Part model, mm, in its own coordinate system. Give positions to 0.01 mm unless a question says otherwise; leave off trailing zeros. Order: outer loops, then holes, each group sorted by start corner. A loop starts at its lowest first (then second) coordinate and runs counter-clockwise, first axis right, second up.
1. Slice it at B-B on z = 14. List the corners of the cut face in (x, y).
2. Drop flat-ended pins along their axis: pin 1 Ø4 at (x, y) = (-5, 2) entering from -Z; pin 2 Ø2 at (y, z) = (5.5, 11) entering from +X; pin 3 Ø1 at (x, z) = (6.5, -16.5) entering from -Y. Give the stop position or say it passes through.
3. Probe line 1 (Z direction, x = 8.5, y = 1.5); line 2 (X direction, y = 9, z = 0.5); line 3 (Z direction, x = -35, y = 1.5). List the from-to ranges inside material, lowest first.
4. Slice it at A-A on y = 2. List the corners of the cut face in (x, z) (1 decimal), and give its area (3 significant figures).
5. Slice it at D-D on x = 26.5. List the corners of the cut face in (y, z), and give its area (3 significant figures).
6. Slice it at C-C on z = -10. List the corners of the cut face in (x, y), and give its area (3 significant figures).
from build123d import *

# Parameters (mm, degrees)
RESSALTO_EXTRUS_O1_DEPTH = 10


with BuildPart() as part:
    # Esboço1 → Ressalto-extrusão1 (new body)
    with BuildSketch(Plane(origin=(0, 0, 0), x_dir=(1, 0, 0), z_dir=(0, 1, 0))):
        with BuildLine():
            ThreePointArc((-39.209518669, -7.912878475), (-38.076880663, -12.253618198), (-36.465309506, -16.440231222))
            ThreePointArc((-36.465309506, -16.440231222), (-33.509440947, -16.163395048), (-31.176914536, -18))
            Line((-31.176914536, -18), (-17.320508076, -10))
            ThreePointArc((-17.320508076, -10), (-17.320508076, 10), (0, 20))
            Line((0, 20), (0, 36))
            ThreePointArc((0, 36), (-2.75680975, 37.101724651), (-3.994996871, 39.8))
            ThreePointArc((-3.994996871, 39.8), (-8.426495684, 39.102355051), (-12.752005558, 37.912878475))
            Line((-12.752005558, 37.912878475), (-39.209518669, -7.912878475))
        make_face()
        with BuildLine():
            Line((-8.660254038, 45), (-12.752005558, 37.912878475))
            ThreePointArc((-12.752005558, 37.912878475), (-8.426495684, 39.102355051), (-3.994996871, 39.8))
            ThreePointArc((-3.994996871, 39.8), (-2.898275349, 42.75680975), (0, 44))
            Line((0, 44), (0, 50))
            ThreePointArc((0, 50), (-5, 48.660254038), (-8.660254038, 45))
        make_face()
        with BuildLine():
            ThreePointArc((8.660254038, 45), (5, 48.660254038), (0, 50))
            Line((0, 50), (0, 44))
            ThreePointArc((0, 44), (2.828427125, 42.828427125), (4, 40))
            ThreePointArc((4, 40), (3.998749022, 39.899968716), (3.994996871, 39.8))
            ThreePointArc((3.994996871, 39.8), (8.426495684, 39.102355051), (12.752005558, 37.912878475))
            Line((12.752005558, 37.912878475), (8.660254038, 45))
        make_face()
        with BuildLine():
            Line((0, 36), (0, 20))
            ThreePointArc((0, 20), (14.142135624, 14.142135624), (20, 0))
            ThreePointArc((20, 0), (19.318516526, -5.176380902), (17.320508076, -10))
            Line((17.320508076, -10), (31.176914536, -18))
            ThreePointArc((31.176914536, -18), (33.509440947, -16.163395048), (36.465309506, -16.440231222))
            ThreePointArc((36.465309506, -16.440231222), (38.076880663, -12.253618198), (39.209518669, -7.912878475))
            Line((39.209518669, -7.912878475), (12.752005558, 37.912878475))
            ThreePointArc((12.752005558, 37.912878475), (8.426495684, 39.102355051), (3.994996871, 39.8))
            ThreePointArc((3.994996871, 39.8), (2.75680975, 37.101724651), (0, 36))
        make_face()
        with BuildLine():
            ThreePointArc((-30.641016151, -20), (-31.127982273, -21.912744878), (-32.470312635, -23.359768778))
            ThreePointArc((-32.470312635, -23.359768778), (-29.65038498, -26.848736852), (-26.457513111, -30))
            Line((-26.457513111, -30), (26.457513111, -30))
            ThreePointArc((26.457513111, -30), (29.65038498, -26.848736852), (32.470312635, -23.359768778))
            ThreePointArc((32.470312635, -23.359768778), (30.752631197, -20.938329603), (31.176914536, -18))
            Line((31.176914536, -18), (17.320508076, -10))
            ThreePointArc((17.320508076, -10), (0, -20), (-17.320508076, -10))
            Line((-17.320508076, -10), (-31.176914536, -18))
            ThreePointArc((-31.176914536, -18), (-30.777312846, -18.96472382), (-30.641016151, -20))
        make_face()
        with BuildLine():
            ThreePointArc((-43.301270189, -15), (-44.641016151, -20), (-43.301270189, -25))
            Line((-43.301270189, -25), (-38.105117767, -22))
            ThreePointArc((-38.105117767, -22), (-38.477621103, -18.868424796), (-36.465309506, -16.440231222))
            ThreePointArc((-36.465309506, -16.440231222), (-38.076880663, -12.253618198), (-39.209518669, -7.912878475))
            Line((-39.209518669, -7.912878475), (-43.301270189, -15))
        make_face()
        with BuildLine():
            Line((-38.105117767, -22), (-43.301270189, -25))
            ThreePointArc((-43.301270189, -25), (-39.641016151, -28.660254038), (-34.641016151, -30))
            Line((-34.641016151, -30), (-26.457513111, -30))
            ThreePointArc((-26.457513111, -30), (-29.65038498, -26.848736852), (-32.470312635, -23.359768778))
            ThreePointArc((-32.470312635, -23.359768778), (-35.579345754, -23.888384955), (-38.105117767, -22))
        make_face()
        with BuildLine():
            Line((38.105117767, -22), (43.301270189, -25))
            ThreePointArc((43.301270189, -25), (44.641016151, -20), (43.301270189, -15))
            Line((43.301270189, -15), (39.209518669, -7.912878475))
            ThreePointArc((39.209518669, -7.912878475), (38.076880663, -12.253618198), (36.465309506, -16.440231222))
            ThreePointArc((36.465309506, -16.440231222), (38.054018746, -17.913995856), (38.641016151, -20))
            ThreePointArc((38.641016151, -20), (38.504719457, -21.03527618), (38.105117767, -22))
        make_face()
        with BuildLine():
            ThreePointArc((32.470312635, -23.359768778), (29.65038498, -26.848736852), (26.457513111, -30))
            Line((26.457513111, -30), (34.641016151, -30))
            ThreePointArc((34.641016151, -30), (39.641016151, -28.660254038), (43.301270189, -25))
            Line((43.301270189, -25), (38.105117767, -22))
            ThreePointArc((38.105117767, -22), (35.579345754, -23.888384955), (32.470312635, -23.359768778))
        make_face()
    extrude(amount=RESSALTO_EXTRUS_O1_DEPTH)


solid = part.part
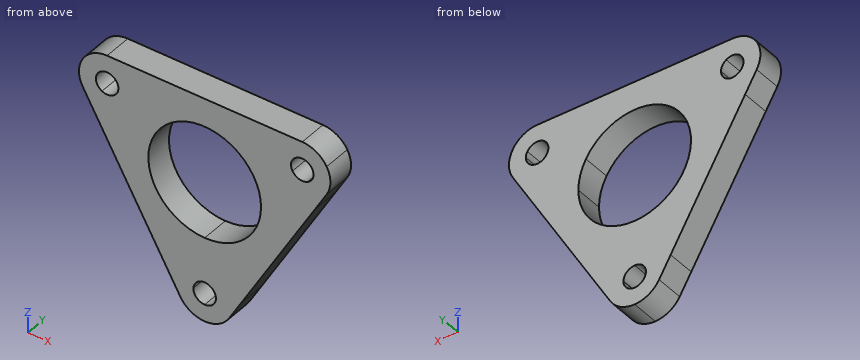
Data:
1. outline: (-42.72, 0) - (-14.28, 0) - (-14.28, 10) - (-42.72, 10) - close; (14.28, 0) - (42.72, 0) - (42.72, 10) - (14.28, 10) - close
2. pin 1: stops at z = -49.54
2. pin 2: stops at x = 41.57
2. pin 3: passes through
3. line 1: z = -45.27 to -18.1, 18.1 to 30
3. line 2: x = -34.93 to -19.99, 19.99 to 34.93
3. line 3: z = 0.62 to 16.02, 23.98 to 29.99
4. outline: (-43.3, 15) - (-8.7, -45) arc R10 ccw to (8.7, -45) - (43.3, 15) arc R10 ccw to (34.6, 30) - (-34.6, 30) arc R10 ccw to start; hole circle Ø8 at (-34.6, 20); hole circle Ø40 at (0, 0); hole circle Ø8 at (0, -40); hole circle Ø8 at (34.6, 20)
4. area: 3,060 mm2
5. outline: (0, -14.1) - (10, -14.1) - (10, 30) - (0, 30) - close
5. area: 441 mm2
6. outline: (-28.87, 0) - (-17.32, 0) - (-17.32, 10) - (-28.87, 10) - close; (17.32, 0) - (28.87, 0) - (28.87, 10) - (17.32, 10) - close
6. area: 231 mm2
